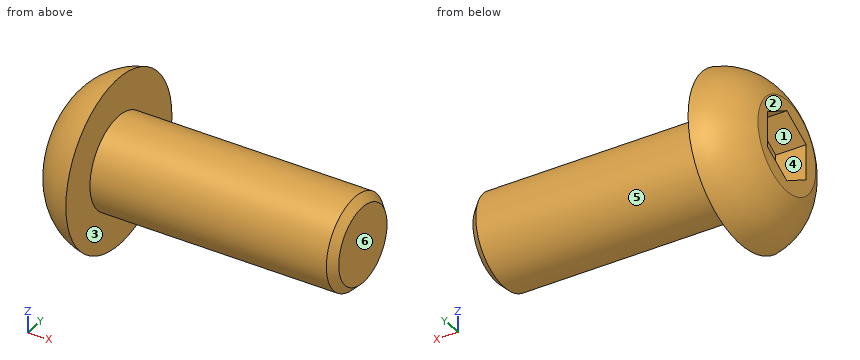
Autodesk Inventor part; units mm, degrees
ref_plane "YZ Plane" through (0, 0, 0) normal (1, 0, 0) x (0, 1, 0)
ref_plane "XZ Plane" through (0, 0, 0) normal (0, 1, 0) x (-1, 0, 0)
ref_plane "XY Plane" through (0, 0, 0) normal (0, 0, 1) x (1, 0, 0)
sketch "Sketch1" plane through (0, 0, 0) normal (0, 0, 1) x (1, 0, 0)
  line L0 (0, 0) -> (9.5, 0)
  line L1 (0, 0) -> (0, 1.5)
  arc A0 (1.5, 2.75) -> (0, 1.5) centre (1.8675, 0.784) ccw
  line L2 (1.5, 2.75) -> (1.5, 1.5)
  line L3 (1.5, 1.5) -> (9.5, 1.5)
  line L4 (9.5, 1.5) -> (9.5, 0)
  dimension "d0" = 1.5
  dimension "d1" = 3
  dimension "d2" = 5.5
  dimension "d3" = 3
  dimension "d4" = 8
  dimension "d5" = 2
revolve "Revolution1" add sketch "Sketch1" angle 360 about axis through (0, 0, 0) along (1, 0, 0)
sketch "Sketch2" plane through (0, 0, 0) normal (-1, 0, 0) x (0, 0, 1)
  line L0 (0.5774, 1) -> (1.1547, 0)
  line L1 (1.1547, 0) -> (0.5774, -1)
  line L2 (0.5774, -1) -> (-0.5774, -1)
  line L3 (-0.5774, -1) -> (-1.1547, 0)
  line L4 (-1.1547, 0) -> (-0.5774, 1)
  line L5 (-0.5774, 1) -> (0.5774, 1)
  point P0 (0, 0)
  point P1 (0, 0)
  dimension "d7" = 2
extrude "Extrusion1" cut sketch "Sketch2" against normal blind 1
thread "Thread1"
chamfer "Chamfer1" distance 0.25 angle 45 1 edges at (9.5, -1.5, 0)
properties part number "M3 X 8mm BHCS"
Verification items for the finished model (mm, model axes). Face numbers are marked on the shaded views. A direction names the side the tool comes from. Give positions to 0.01 mm unless a question says otherwise; leave off trailing zeros. Order: outer loops, then holes, each group sorted by start corner. A loop starts at its lowest first (then second) coordinate and runs counter-clockwise, first axis right, second up. Notation, with made-up numbers: (-16.5, 19.25) -> (21.5, 19.25) arc R35 cw to (21.5, 56.25) -> close; hole circle Ø10 at (54, 46). An arc over 180 degrees is marked (long way). One line per item, written item: value.
(1) Tool access check on the marked faces 1, 2 and 3. Record the directions out of +Z, -Z, +X, -X, +Y, -Y that give a thin tool (end or side, any length) a straight path to the whole face; none if there is none.
Final values:
face 1: -X
face 2: +Z, -Z, -X, +Y, -Y
face 3: +X
(2) Scan lines: line 1 along X through (y, z) = (0.65, 0.55); line 2 along X through (y, z) = (2.3, -0.95); line 3 along Y through (x, z) = (6.5, 0.4). Record each from-to range of solid material in increasing order. Write a range as [from, to].
Final values:
line 1: [1, 9.5]
line 2: [0.82, 1.5]
line 3: [-1.45, 1.45]
(3) Draft check along Z on the marked faces 4, 5 and 6. Enter one of: pulls with the +Z half, pulls with the -Z half, needs draft (parallel to the pull), parting line crosses it, or undercut.
Final values:
face 4: undercut
face 5: parting line crosses it
face 6: needs draft
(4) Gauge pin test, flat ends, axial feed: pin 1 (1 mm diameter, centred on y = 1, z = 1, fed in from +X); pin 2 (1.1 mm diameter, centred on x = 0.5, z = 0, fed in from -Y); pin 3 (0.5 mm diameter, centred on x = 0.5, z = -0.5, fed in from +Y); pin 4 (2 mm diameter, centred on x = 8, y = -1, fed in from -Z). Record the tip position at first contact, or that the pin passes through.
Final values:
pin 1: x = 9.5
pin 2: y = -2.61
pin 3: y = 2.4
pin 4: z = -1.5
(5) Sectioned sample at A-A on x = 7. Record the cut outline in (y, z), then the cut area to 3 significant figures.
Final values:
outline: circle Ø3 at (0, 0)
area: 7.07 mm^2
